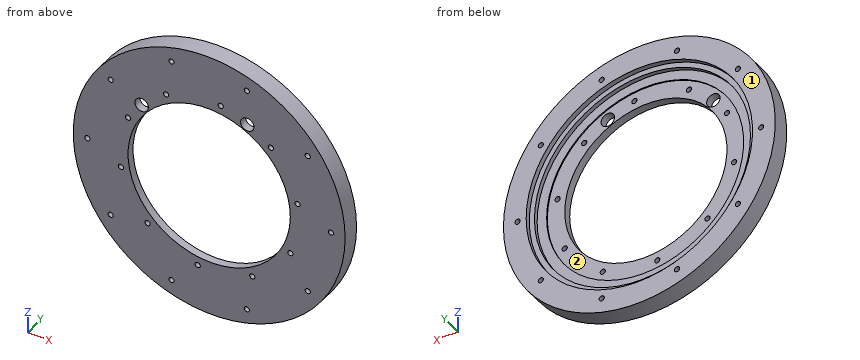
Autodesk Inventor part; units mm, degrees
ref_plane "Work Plane1" through (3.7155, 65.557, 54.6036) normal (0, -1, 0) x (0.9033475, 0, -0.4289095)
ref_plane "Work Plane2" through (-48.1402, 113.182, 79.2247) normal (0, 0, 1) x (1, 0, 0)
ref_plane "Work Plane3" through (-48.1402, 113.182, 79.2247) normal (0, 0, 1) x (1, 0, 0)
ref_plane "Work Plane1" through (3.7155, 65.557, 54.6036) normal (0, -1, 0) x (0.9033475, 0, -0.4289095)
sketch "Sketch2" plane through (3.7155, 65.557, 54.6036) normal (0, -1, 0) x (0.9033475, 0, -0.4289095)
  circle A0 centre (-118.0349, 16.246) radius 4.7625
  circle A1 centre (-57.404, 62.7698) radius 4.7625
  circle A2 centre (-57.404, 0) radius 69.723
  circle A3 centre (-57.404, 0) radius 57.404
  circle A4 centre (-57.404, 0) radius 76.2
  circle A5 centre (-57.404, 0) radius 84.2
  circle A6 centre (-107.7614, 37.4723) radius 1.0795
  circle A7 centre (-50.1308, 62.3469) radius 1.0795
  circle A8 centre (0.2267, 24.8747) radius 1.0795
  circle A9 centre (-7.0466, -37.4723) radius 1.0795
  circle A10 centre (-64.6772, -62.3469) radius 1.0795
  circle A11 centre (-115.0347, -24.8747) radius 1.0795
  circle A12 centre (-19.0569, -49.9749) radius 1.6475
  circle A13 centre (-95.7511, 49.9749) radius 1.651
  circle A14 centre (-120.1738, 0) radius 4.7625
  circle A15 centre (-41.158, 60.6309) radius 4.7625
  point P0 (20.0636, -50.9196)
  dimension "d0" = 8
extrude "Extrusion1" [suppressed]
ref_plane "Work Plane2" through (-48.1402, 113.182, 79.2247) normal (0, 0, 1) x (1, 0, 0)
sketch "Sketch4" plane through (-48.1402, 113.182, 79.2247) normal (0, 0, 1) x (1, 0, 0)
  line L0 (-76.2, -47.625) -> (76.2, -47.625) construction
  line L1 (0, -48.4188) -> (0, 19.2501)
  line L2 (-57.404, -47.625) -> (57.404, -47.625) construction
  line L3 (57.404, -47.625) -> (57.404, -48.4188)
  line L4 (57.404, -48.4188) -> (69.723, -48.4188)
  line L5 (69.723, -47.625) -> (-69.723, -47.625) construction
  line L6 (69.723, -48.4188) -> (69.723, -47.625)
  line L7 (69.723, -47.625) -> (76.2, -47.625)
  line L8 (76.2, -47.625) -> (76.2, -41.2188) construction
  line L9 (76.2, -41.2188) -> (96.2, -41.2188) construction
  line L10 (96.2, -41.2188) -> (96.2, -53.9188)
  line L11 (96.2, -53.9188) -> (57.404, -53.9188)
  line L12 (57.404, -53.9188) -> (57.404, -48.4188)
  line L13 (76.2, -44.6478) -> (80.1116, -44.6478)
  line L14 (80.1116, -44.6478) -> (80.1116, -41.2188)
  line L15 (80.1116, -41.2188) -> (76.2, -41.2188) construction
  line L16 (76.2, -41.2188) -> (76.2, -44.6478) construction
  line L17 (76.2, -44.6478) -> (76.2, -47.625)
  line L18 (76.2, -41.2188) -> (76.2, -41.2188) construction
  line L19 (96.2, -41.2188) -> (80.1116, -41.2188)
  point P0 (48.1402, -113.182)
  dimension "d4" = 20
  dimension "d9" = 3.9116
  dimension "d10" = 3.429
  dimension "d14" = 12.7
  dimension "d15" = 5.5
  dimension "d32" = 0.7937
revolve "Revolution1" add sketch "Sketch4" angle 360 about axis through (-48.1402, 64.7633, 79.2247) along (0, 1, 0) separate body
sketch "Sketch5" plane through (-48.1402, 59.2633, 79.2247) normal (0, -1, 0) x (1, 0, 0)
  circle A0 centre (0, 0) radius 57.404
  circle A1 centre (26.9225, 56.7029) radius 4.7625
  circle A2 centre (40.681, 47.8027) radius 4.7625
  circle A3 centre (-56.7029, 26.9225) radius 4.7625
  circle A4 centre (-47.8027, 40.681) radius 4.7625
  circle A5 centre (0, 0) radius 69.723
  point P0 (48.1402, -79.2247)
extrude "Extrusion2" cut sketch "Sketch5" against normal through all contours A1 | A4
ref_plane "Work Plane3" through (-48.1402, 113.182, 79.2247) normal (0, 0, 1) x (1, 0, 0)
sketch "Sketch8" plane through (-48.1402, 71.9633, 79.2247) normal (0, 1, 0) x (1, 0, 0)
  circle A0 centre (0, 0) radius 96.2
  line L0 (96.2, 0) -> (76.2, 0)
  circle A1 centre (0, 0) radius 76.2
  point P0 (48.1402, 79.2247)
  point P1 (86.2, 0)
  dimension "d39" = 152.4
hole "Hole1" at (38.0598, 71.9633, 79.2247) direction (0, -1, 0) diameter 3.683 end through all
pattern_circular "Circular Pattern1" count 10 over 360 about axis through (-48.1402, 65.6133, 79.2247) along (0, -1, 0) of "Hole1"
sketch "Sketch12" plane through (-48.1402, 64.7633, 79.2247) normal (0, -1, 0) x (1, 0, 0)
  circle A0 centre (-62.4688, -11.7461) radius 1.8415
  circle A1 centre (-30.4751, 55.7816) radius 1.8415
  circle A2 centre (62.4688, 11.7461) radius 1.8415
  circle A3 centre (30.4751, -55.7816) radius 1.8415
  circle A4 centre (8.1327, 63.0411) radius 1.8415
  circle A5 centre (-8.1327, -63.0411) radius 1.8415
  circle A6 centre (57.4425, -27.2155) radius 1.8415
  circle A7 centre (43.6341, 46.221) radius 1.8415
  circle A8 centre (-57.4425, 27.2155) radius 1.8415
  circle A9 centre (-43.6341, -46.221) radius 1.8415
  circle A10 centre (0, 0) radius 57.404
  circle A11 centre (0, 0) radius 72.898
  circle A12 centre (26.9225, 56.7029) radius 4.7625
  circle A13 centre (-47.8027, 40.681) radius 4.7625
  circle A14 centre (0, 0) radius 57.404
  circle A15 centre (0, 0) radius 69.723
  point P0 (48.1402, -79.2247)
extrude "Extrusion6" cut sketch "Sketch12" along normal through all contours A0 | A1 | A2 | A3 | A4 | A5 | A6 | A7 | A8 | A9
sketch "Sketch13" plane through (-48.1402, 71.9633, 79.2247) normal (0, 1, 0) x (1, 0, 0)
  circle A0 centre (0, 0) radius 96.2
  circle A1 centre (0, 0) radius 76.454
  point P0 (48.1402, 79.2247)
  dimension "d35" = 152.908
extrude "Extrusion7" cut sketch "Sketch13" against normal up to surface (6.4063 mm away) contours A1
properties part number "1133_RU End Cap"
Geometry check sheet. Reference: the model listing, model coordinates, mm. Face numbers are marked on the shaded views. Coordinates: 2 decimals unless noted, no trailing zeros. Order: outer loops, then holes, each group sorted by start corner. A loop starts at its lowest first (then second) coordinate and runs counter-clockwise, first axis right, second up.
Item 1: Section check A-A (x = -32.5). Enter the section's corners in (y, z).
Item 2: Depth check by flat-ended pin: pin 1 (5 mm diameter, centred on x = 9.3, z = 52.01, fed in from +Y); pin 2 (3 mm diameter, centred on x = -83, y = 61.5, fed in from -Z); pin 3 (3 mm diameter, centred on x = -103.5, y = 70.5, fed in from -Z). Enter the tip coordinate at first touch or a pass-through.
Item 3: Mould release check, pull along X, two halves, no side actions. Record for the marked faces 1 and 2: released by +X, released by -X, zero draft, split by the parting line, or undercut.
Item 4: Section check B-B (z = 38). Enter the section's corners in (x, y), plus the area to 3 significant figures.
Item 5: Scan lines: line 1 along X through (y, z) = (61.5, 79.5); line 2 along X through (y, z) = (61.75, 89.5); line 3 along Z through (x, y) = (-46, 66.5). Record each from-to range of solid material in increasing order.
Check sheet entries:
1. outline: (59.26, -15.7) - (71.96, -15.7) - (71.96, 0.65) - (68.53, 0.65) - (68.53, 4.39) - (65.56, 4.39) - (65.56, 11.28) - (64.76, 11.28) - (64.76, 23.99) - (59.26, 23.99) - close; (59.26, 134.46) - (64.76, 134.46) - (64.76, 147.17) - (65.56, 147.17) - (65.56, 154.06) - (68.53, 154.06) - (68.53, 157.79) - (71.96, 157.79) - (71.96, 174.14) - (59.26, 174.14) - close
2. pin 1: stops at y = 64.76
2. pin 2: stops at z = -11.01
2. pin 3: stops at z = -0.48
3. face 1: zero draft
3. face 2: undercut
4. outline: (-135.06, 59.26) - (-88.09, 59.26) - (-88.09, 64.76) - (-104.37, 64.76) - (-104.37, 65.56) - (-112.53, 65.56) - (-112.53, 68.53) - (-116.83, 68.53) - (-116.83, 71.96) - (-135.06, 71.96) - close; (-8.19, 59.26) - (38.78, 59.26) - (38.78, 71.96) - (20.55, 71.96) - (20.55, 68.53) - (16.25, 68.53) - (16.25, 65.56) - (8.09, 65.56) - (8.09, 64.76) - (-8.19, 64.76) - close
4. area: 825 mm2
5. line 1: x = -144.34 to -136.16, -132.52 to -105.54, 9.26 to 36.24, 39.88 to 48.06
5. line 2: x = -143.79 to -104.62, 8.34 to 13.22, 15.44 to 47.51
5. line 3: z = -16.95 to 2.8, 155.65 to 175.4
